Read the model definition and answer for the solid it produces. Units are mm, in the model's axes. Coordinates: 2 decimals unless noted, no trailing zeros. Loops run counter-clockwise (first coordinate to the right, second up) from the corner with the lowest first, then second, coordinate; pieces in that order, holes last. Notation, with made-up numbers: (2, 85.5) - (18, 85.5) arc R24 cw to (18, 100.5) - close; hole circle Ø7 at (33.25, -9.75). An arc over 180 degrees is marked (long way). Use one line per item in the form item = value. Start each with the question number.
1) A cutting plane is placed at C-C (z = -65). Give the vertices of the cut face in (x, y), and give its area (3 significant figures).
2) A cutting plane is placed at D-D (y = 2.15). State how many separate pieces and enclosed holes the cut face has, and give its area (3 significant figures).
3) The mould has two halves that part along X. Classify faces 1 (the face through (-19, 3, 18)), 2 (the face through (-31.6, 1.5, -20.9)): released by +X, released by -X, zero draft, split by the parting line, or undercut.
4) Consider line 1 (X direction, y = 1, z = -69); line 2 (X direction, y = 1.65, z = -62.5); line 3 (Z direction, x = 61, y = 2.8). Determine where each line is inside the solid, lowest interval first.
5) Each of these flat-tipped pins is pushed along its axis until it touches: P1, Ø1.8, axis at x = 0, z = 130, coming from the +Y side; P2, Ø1.5, axis at y = 1.5, z = -87, coming from the -X side; P3, Ø1.5, axis at y = 1.5, z = 71, coming from the +X side. Where does it stop, or does it pass through?
6) A cutting plane is placed at B-B (x = -25.5). Give the vertices of the cut face in (y, z), and give its area (3 significant figures).
7) A cutting plane is placed at A-A (z = 58). Give the vertices of the cut face in (x, y).
from build123d import *

# Parameters (mm, degrees)
SKETCH1_W           = 160
SKETCH1_H           = 260
BOSS_EXTRUDE1_DEPTH = 3
SKETCH2_R           = 1.5
SKETCH2_R_2         = 8
SKETCH2_R_3         = 27.5
CUT_EXTRUDE1_DEPTH  = 3
SKETCH7_W           = 3
SKETCH7_H           = 3
SKETCH7_W_2         = 10
SKETCH7_H_2         = 10
CUT_EXTRUDE2_DEPTH  = 171.026468528


with BuildPart() as part:
    # Sketch1 → Boss-Extrude1 (new body)
    with BuildSketch(Plane(origin=(0, 0, 0), x_dir=(1, 0, 0), z_dir=(0, 1, 0))):
        with Locations((0, -20)):
            Rectangle(SKETCH1_W, SKETCH1_H)
    extrude(amount=BOSS_EXTRUDE1_DEPTH)

    # Sketch2 → Cut-Extrude1 (cut)
    with BuildSketch(Plane(origin=(0, 3, 0), x_dir=(1, 0, 0), z_dir=(0, 1, 0))):
        with Locations(Location((0, -10, 0), (0, 0, 270))):
            Circle(SKETCH2_R)
        with Locations(Location((0, -130, 0), (0, 0, 270))):
            Circle(SKETCH2_R)
        with Locations(Location((-37, 15, 0), (0, 0, 270))):
            Circle(SKETCH2_R_2)
        with Locations(Location((-12.75, 93.25, 0), (0, 0, 270))):
            Circle(SKETCH2_R)
        with Locations(Location((37, 15, 0), (0, 0, 90))):
            Circle(SKETCH2_R_2)
        with Locations(Location((-12.75, 44.75, 0), (0, 0, 270))):
            Circle(SKETCH2_R)
        with Locations(Location((-61.25, 44.75, 0), (0, 0, 270))):
            Circle(SKETCH2_R)
        with Locations(Location((-61.25, 93.25, 0), (0, 0, 270))):
            Circle(SKETCH2_R)
        with Locations(Location((37, 69, 0), (0, 0, 90))):
            Circle(SKETCH2_R_3)
        with Locations(Location((12.75, 44.75, 0), (0, 0, 90))):
            Circle(SKETCH2_R)
        with Locations(Location((61.25, 44.75, 0), (0, 0, 90))):
            Circle(SKETCH2_R)
        with Locations(Location((61.25, 93.25, 0), (0, 0, 90))):
            Circle(SKETCH2_R)
        with Locations(Location((-37, 69, 0), (0, 0, 270))):
            Circle(SKETCH2_R_3)
        with Locations(Location((12.75, 93.25, 0), (0, 0, 90))):
            Circle(SKETCH2_R)
        with BuildLine():
            Line((1.5, -15), (1.5, -125))
            ThreePointArc((1.5, -125), (0, -126.5), (-1.5, -125))
            Line((-1.5, -125), (-1.5, -15))
            ThreePointArc((-1.5, -15), (0, -13.5), (1.5, -15))
        make_face()
    extrude(amount=-CUT_EXTRUDE1_DEPTH, mode=Mode.SUBTRACT)

    # Sketch7 → Cut-Extrude2 (cut, through all)
    with BuildSketch(Plane(origin=(0, 3, 0), x_dir=(1, 0, 0), z_dir=(0, 1, 0))):
        with Locations((0, 108.5)):
            Rectangle(SKETCH7_W, SKETCH7_H)
        with Locations((40, 108.5)):
            Rectangle(SKETCH7_W_2, SKETCH7_H)
        with Locations((-40, 108.5)):
            Rectangle(SKETCH7_W_2, SKETCH7_H)
        with Locations((40, -148.5)):
            Rectangle(SKETCH7_W_2, SKETCH7_H)
        with Locations((-40, -148.5)):
            Rectangle(SKETCH7_W_2, SKETCH7_H)
        with Locations((0, -148.5)):
            Rectangle(SKETCH7_W, SKETCH7_H)
        with Locations((-78.5, -125)):
            Rectangle(SKETCH7_W, SKETCH7_H_2)
        with Locations((-78.5, -20)):
            Rectangle(SKETCH7_W, SKETCH7_H_2)
        with Locations((-78.5, 85)):
            Rectangle(SKETCH7_W, SKETCH7_H_2)
        with Locations((-78.5, -71.5)):
            Rectangle(SKETCH7_W, SKETCH7_H)
        with Locations((-78.5, 31.5)):
            Rectangle(SKETCH7_W, SKETCH7_H)
        with Locations((78.5, -125)):
            Rectangle(SKETCH7_W, SKETCH7_H_2)
        with Locations((78.5, -71.5)):
            Rectangle(SKETCH7_W, SKETCH7_H)
        with Locations((78.5, -20)):
            Rectangle(SKETCH7_W, SKETCH7_H_2)
        with Locations((78.5, 31.5)):
            Rectangle(SKETCH7_W, SKETCH7_H)
        with Locations((78.5, 85)):
            Rectangle(SKETCH7_W, SKETCH7_H_2)
    extrude(amount=-CUT_EXTRUDE2_DEPTH, mode=Mode.SUBTRACT)


solid = part.part
Found:
q1.outline = (-80, 0) - (-64.21, 0) - (-64.21, 3) - (-80, 3) - close; (-9.79, 0) - (9.79, 0) - (9.79, 3) - (-9.79, 3) - close; (64.21, 0) - (80, 0) - (80, 3) - (64.21, 3) - close
q1.area = 154 mm^2
q2.separate_pieces = 1
q2.enclosed_holes = 15
q2.area = 35,700 mm^2
q3.face_1 = zero draft
q3.face_2 = undercut
q4.line_1 = -80 to -64.5, -9.5 to 9.5, 64.5 to 80
q4.line_2 = -80 to -63.72, -10.28 to 10.28, 63.72 to 80
q4.line_3 = -110 to -94.73, -91.77 to -82.43, -55.57 to -46.23, -43.27 to 150
q5.P1 = through
q5.P2 = -77
q5.P3 = 77
q6.outline = (0, -110) - (3, -110) - (3, -93.98) - (0, -93.98) - close; (0, -44.02) - (3, -44.02) - (3, 150) - (0, 150) - close
q6.area = 630 mm^2
q7.outline = (-80, 0) - (-1.5, 0) - (-1.5, 3) - (-80, 3) - close; (1.5, 0) - (80, 0) - (80, 3) - (1.5, 3) - close
